from build123d import *


with BuildPart() as part:
    # Sketch1 → Loft1 section 0
    with BuildSketch(Plane(origin=(0, 0, 0), x_dir=(1, 0, 0), z_dir=(0, 1, 0)), mode=Mode.PRIVATE) as loft1_s0:
        Polygon((5.410441731, -1.234898019), (4.338837391, 3.460107358), (0, 5.549581321), (-4.338837391, 3.460107358), (-5.410441731, -1.234898019), (-2.407873094, -5), (2.407873094, -5), align=None)
    loft([Vertex(0, 20, 0), loft1_s0.sketch])


solid = part.part
Model file for the job. Use its own axes, mm. Coordinates: 2 decimals unless noted, no trailing zeros. Order: outer loops, then holes, each group sorted by start corner. A loop starts at its lowest first (then second) coordinate and runs counter-clockwise, first axis right, second up. Notation, with made-up numbers: (-2, 62.25) -> (52, 62.25) arc R21 cw to (52, 99.25) -> close; hole circle Ø4 at (81.25, 42.5). An arc over 180 degrees is marked (long way). Return JSON: item names as keys, results as strings. Group by question number.
Item 1: Saw through at B-B on x = 1.5. Write the cut outline in (y, z).
Item 2: Wall check: line 1 along Z through (x, y) = (3.5, 3.25); line 2 along Z through (x, y) = (0.5, 1.75); line 3 along X through (y, z) = (18, 0). Give the ranges that are in metal, low to high. Write a range as [from, to].
Item 3: Saw through at C-C on z = -2.75. Write the cut outline in (x, y).
Item 4: Flat gauge pins, fed straight in: P1, Ø6, axis at y = 6.5, z = -1.5, coming from the +X side; P2, Ø1.5, axis at y = 15.5, z = 3, coming from the -X side; P3, Ø1.5, axis at x = -3.5, y = 4, coming from the +Z side; P4, Ø1, axis at y = 2.5, z = 3, coming from the -X side. Where does each tip first touch, or does it go through?
Item 5: Saw through at A-A on y = 3.5. Write the cut outline in (x, z) (1 decimal), then the cut area to 3 significant figures.
Item 6: Saw through at D-D on y = 16. Write the cut outline in (x, z).
Values found:
{
 "1": {"outline": "(0, -4.83) -> (13.09, -1.2) -> (14.46, 0.34) -> (7.54, 3.11) -> (0, 5) -> close"},
 "2": {"line 1": "z = [-2.96, 2.33]", "line 2": "z = [-4.82, 4.56]", "line 3": "x = [-0.51, 0.51]"},
 "3": {"outline": "(-4.5, 0) -> (4.5, 0) -> (3.45, 4.1) -> (0, 10.09) -> (-3.45, 4.1) -> close"},
 "4": {"P1": "stops at x = 4.15", "P2": "passes through", "P3": "stops at z = 3.01", "P4": "stops at x = -3.63"},
 "5": {"outline": "(-4.5, 1) -> (-3.6, -2.9) -> (0, -4.6) -> (3.6, -2.9) -> (4.5, 1) -> (2, 4.1) -> (-2, 4.1) -> close", "area": "57.4 mm2"},
 "6": {"outline": "(-1.08, 0.25) -> (-0.87, -0.69) -> (0, -1.11) -> (0.87, -0.69) -> (1.08, 0.25) -> (0.48, 1) -> (-0.48, 1) -> close"}
}
